Could you check a few things on this drawing? It's one solid part, dimensions in mm from its lowest x, y, z. Give positions to 0.01 mm unless a question says otherwise; leave off trailing zeros. Loops run counter-clockwise (first coordinate to the right, second up) from the corner with the lowest first, then second, coordinate; pieces in that order, holes last. Notation, with made-up numbers: (-11.5, 25) - (-5.5, 25) arc R12 cw to (-5.5, 41) - close; hole circle Ø6 at (75, 50). An arc over 180 degrees is marked (long way). Write item = value, one per line.
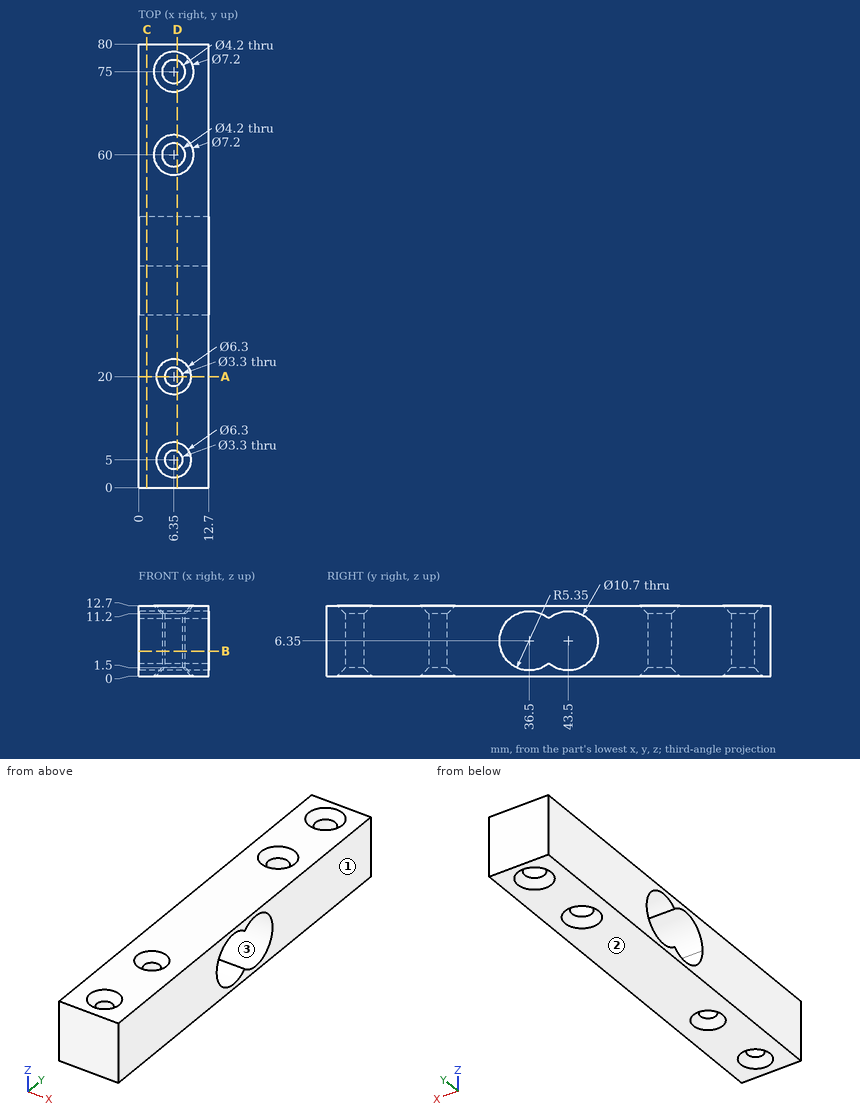
Q1. Imagine slicing it at D-D, the plane x = 7. Give the number of separate pieces and of enclosed holes in the cut face, then the cut area to 3 significant figures.
Output:
separate_pieces = 5
enclosed_holes = 1
area = 660 mm2
Q2. For pin 1 (4 mm diameter, centred on x = 6.35, y = 75, fed in from -Z); pin 2 (6.5 mm diameter, centred on x = 6.35, y = 60, fed in from +Z), each with a flat end and sliding along its axis, tell me the tip position at first contact or that it passes through.
Output:
pin_1 = through
pin_2 = 12.35
Q3. Imagine slicing it at A-A, the plane y = 20. Write out the boundary of the cut face in (x, z).
Output:
outline = (0, 0) - (3.2, 0) - (4.7, 1.5) - (4.7, 11.2) - (3.2, 12.7) - (0, 12.7) - close; (8, 1.5) - (9.5, 0) - (12.7, 0) - (12.7, 12.7) - (9.5, 12.7) - (8, 11.2) - close
Q4. Imagine slicing it at C-C, the plane x = 1.5. Write out the boundary of the cut face in (y, z), then the cut area to 3 significant figures.
Output:
outline = (0, 0) - (80, 0) - (80, 12.7) - (0, 12.7) - close; hole (40, 2.3) arc R5.35 ccw (long way) to (40, 10.4) arc R5.35 ccw (long way) to start
area = 857 mm2
Q5. I need wall thicknesses on L1, parallel to Y at x = 6.35, z = 6.5; L2, parallel to Z at x = 6.25, y = 43.5; L3, parallel to Y at x = 9.5, z = 10.75. Which ranges of each line are inside material? Lowest first, please.
Output:
L1 = 0 to 3.35, 6.65 to 18.35, 21.65 to 31.15, 48.85 to 57.9, 62.1 to 72.9, 77.1 to 80
L2 = 0 to 1, 11.7 to 12.7
L3 = 0 to 33.46, 39.54 to 40.46, 46.54 to 80
Q6. We'd pull the mould along Z, two halves only. Please class the marked faces 1, 2 and 3: released by +Z, released by -Z, zero draft, split by the parting line, or undercut.
Output:
face_1 = zero draft
face_2 = released by -Z
face_3 = undercut
Q7. Imagine slicing it at B-B, the plane z = 4.5. Write out the boundary of the cut face in (x, y), then the cut area to 3 significant figures.
Output:
outline = (0, 0) - (12.7, 0) - (12.7, 31.48) - (0, 31.48) - close; (0, 48.52) - (12.7, 48.52) - (12.7, 80) - (0, 80) - close; hole circle Ø4.2 at (6.35, 60); hole circle Ø4.2 at (6.35, 75); hole circle Ø3.3 at (6.35, 5); hole circle Ø3.3 at (6.35, 20)
area = 755 mm2
